Study the drawing (mm; zero at the part's minimum x, y, z) and answer. A direction names the side the tool comes from. Coordinates: 2 decimals unless noted, no trailing zeros. Order: outer loops, then holes, each group sorted by start corner. A loop starts at its lowest first (then second) coordinate and runs counter-clockwise, first axis right, second up. Notation, with made-up numbers: (-7, 81.5) -> (36, 81.5) arc R15 cw to (36, 110.5) -> close; hole circle Ø7 at (61.25, -32.5). An arc over 180 degrees is marked (long way). Write each question's results on one line, items separated by ' | '. Start each with the question number.
(1) Given pin 1 (11.5 mm diameter, centred on x = 7.32, y = 20.81, fed in from -Z); pin 2 (5 mm diameter, centred on x = 23.5, y = 9.5, fed in from -Z); pin 3 (2 mm diameter, centred on x = 10.5, z = 4.5, fed in from -Y), each flat-ended and moving along its own axis, determine where each tip first touches the part or whether it passes through.
(2) The part is cut by section A-A, the plane z = 1.8. Give the vertices of the cut face in (x, y).
(3) The part is cut by section C-C, the plane y = 17.5. Give the vertices of the cut face in (x, z).
(4) Determine the mould class of the marked faces 3, 4 and 5 for opening direction X: +X half, -X half, draft (parallel to the pull), parting line (faces both ways), or undercut.
(5) The part is cut by section B-B, the plane x = 17.5. Give the vertices of the cut face in (y, z).
(6) Straight lines are drawn through the part: L1, parallel to Y at x = 17.5, z = 2.45; L2, parallel to Y at x = 13.5, z = 3.1 (1 decimal); L3, parallel to Y at x = 7, z = 3.65 (1 decimal). For each, find the intervals that lie inside material, in ascending order.
(7) A tool of negligible diameter and unlimited length cuts with its end or side. For the marked faces 1 and 2, from which of +Z, -Z, +X, -X, +Y, -Y can it reach the whole face along a straight path? Write none if from no direction.
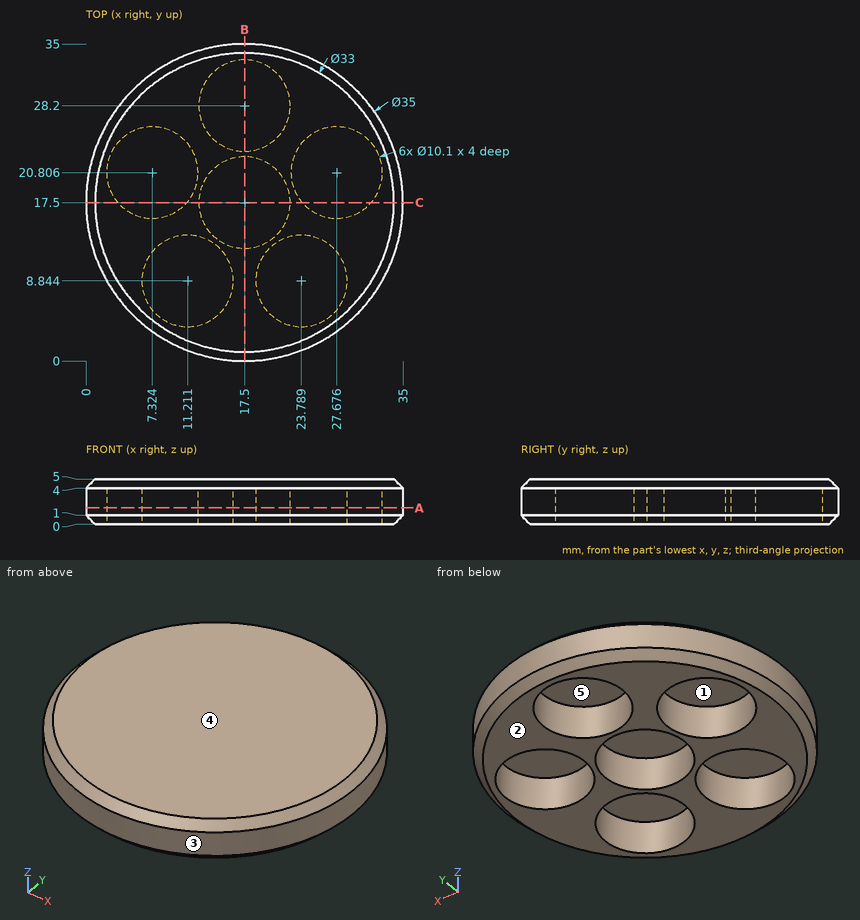
Established:
1) pin 1: stops at z = 0 | pin 2: stops at z = 4 | pin 3: stops at y = 1.11
2) outline: circle Ø35 at (17.5, 17.5); hole circle Ø10.1 at (7.32, 20.81); hole circle Ø10.1 at (11.21, 8.84); hole circle Ø10.1 at (17.5, 17.5); hole circle Ø10.1 at (17.5, 28.2); hole circle Ø10.1 at (23.79, 8.84); hole circle Ø10.1 at (27.68, 20.81)
3) outline: (0, 1) -> (1, 0) -> (3.51, 0) -> (3.51, 4) -> (11.14, 4) -> (11.14, 0) -> (12.45, 0) -> (12.45, 4) -> (22.55, 4) -> (22.55, 0) -> (23.86, 0) -> (23.86, 4) -> (31.49, 4) -> (31.49, 0) -> (34, 0) -> (35, 1) -> (35, 4) -> (34, 5) -> (1, 5) -> (0, 4) -> close
4) face 3: parting line | face 4: draft | face 5: undercut
5) outline: (0, 1) -> (1, 0) -> (12.45, 0) -> (12.45, 4) -> (22.55, 4) -> (22.55, 0) -> (23.15, 0) -> (23.15, 4) -> (33.25, 4) -> (33.25, 0) -> (34, 0) -> (35, 1) -> (35, 4) -> (34, 5) -> (1, 5) -> (0, 4) -> close
6) L1: y = 0 to 12.45, 22.55 to 23.15, 33.25 to 35 | L2: y = 0.5 to 4.3, 13.3 to 14.4, 20.6 to 25.1, 31.3 to 34.5 | L3: y = 3.5 to 6.1, 11.6 to 15.8, 25.8 to 31.5
7) face 1: -Z | face 2: -Z, +X, -X, +Y, -Y
